from build123d import *

# Parameters (mm, degrees)
BASPROSKE_W         = 3
BASPROSKE_H         = 24.5
TOOTHCUT_DEPTH      = 35.777866525
TEETHCUTS_COUNT     = 26
TEETHCUTS_ANGLE     = 346.153846154
BORSKE_R            = 3
BORE_DEPTH          = 50.0000508
BOSS_EXTRUDE1_START = 3
SKETCH1_R           = 2.770499524
SKETCH1_R_2         = 3
BOSS_EXTRUDE1_DEPTH = 3


with BuildPart() as part:
    # BasProSke → Base-Revolve (revolve)
    with BuildSketch(Plane(origin=(0, 0, 0), x_dir=(1, 0, 0), z_dir=(0, 1, 0)), mode=Mode.PRIVATE) as base_revolve_sk:
        with Locations((1.5, 12.25)):
            Rectangle(BASPROSKE_W, BASPROSKE_H)
    revolve(base_revolve_sk.sketch.rotate(Axis((-10, 0, 0), (1, 0, 0)), 180), axis=Axis((-10, 0, 0), (1, 0, 0)))

    # TooCutSke → ToothCut (cut, through all)
    with BuildSketch(Plane(origin=(0, 0, 0), x_dir=(0, 0, -1), z_dir=(1, 0, 0))):
        with BuildLine():
            ThreePointArc((0.813448928, 20.545402967), (0, 20.5615), (-0.813448928, 20.545402967))
            ThreePointArc((-0.813448928, 20.545402967), (-1.408477569, 22.569593712), (-2.4536582, 24.402352481))
            ThreePointArc((-2.4536582, 24.402352481), (0, 24.5254), (2.4536582, 24.402352481))
            ThreePointArc((2.4536582, 24.402352481), (1.408477569, 22.569593712), (0.813448928, 20.545402967))
        make_face()
    toothcut = extrude(amount=TOOTHCUT_DEPTH, mode=Mode.SUBTRACT)

    # TeethCuts: ToothCut ×26 about axis
    teethcuts_axis = Axis((-10, 0, 0), (1, 0, 0))
    for i in range(1, TEETHCUTS_COUNT):
        add(toothcut.rotate(teethcuts_axis, i * TEETHCUTS_ANGLE / (TEETHCUTS_COUNT - 1)), mode=Mode.SUBTRACT)

    # BorSke → Bore (cut, symmetric)
    with BuildSketch(Plane(origin=(0, 0, 0), x_dir=(0, 0, -1), z_dir=(1, 0, 0))):
        with Locations(Location((0, 0, 0), (0, 0, 180))):
            Circle(BORSKE_R)
    extrude(amount=BORE_DEPTH, both=True, mode=Mode.SUBTRACT)

    # Sketch1 → Boss-Extrude1 (add)
    with BuildSketch(Plane(origin=(0, 0, 0), x_dir=(0, 0, -1), z_dir=(1, 0, 0)).offset(BOSS_EXTRUDE1_START)):
        with BuildLine():
            Line((-0.723220082, -5.956253245), (-54.329499283, 0.552727489))
            ThreePointArc((-54.329499283, 0.552727489), (-59.562532446, 7.232200815), (-52.88305912, 12.465233978))
            Line((-52.88305912, 12.465233978), (0.723220082, 5.956253245))
            ThreePointArc((0.723220082, 5.956253245), (5.956253245, -0.723220082), (-0.723220082, -5.956253245))
        make_face()
        with Locations((-53.606279201, 6.508980734)):
            Circle(SKETCH1_R, mode=Mode.SUBTRACT)
        with Locations(Location((0, 0, 0), (0, 0, 180))):
            Circle(SKETCH1_R_2, mode=Mode.SUBTRACT)
    extrude(amount=-BOSS_EXTRUDE1_DEPTH)


solid = part.part
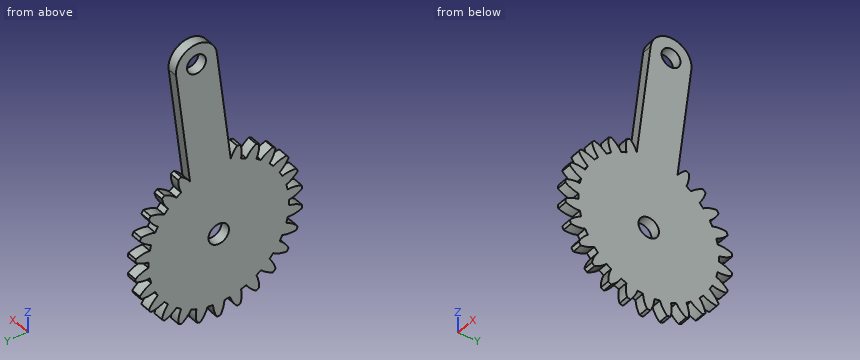
The listing builds one solid part. Answer for the finished solid, in the listing's coordinates (mm). Coordinates: 2 decimals unless noted, no trailing zeros. Write each loop counter-clockwise with the first axis right and the second up, starting at its lowest first coordinate (ties: lowest second). Pieces come first, ordered by that corner, then holes. Notation, with made-up numbers: (5, 18) - (54, 18) arc R32 cw to (54, 55) - close; hole circle Ø4 at (-13, 47.25). An arc over 180 degrees is marked (long way). Return JSON: item names as keys, results as strings.
1. Each of these flat-tipped pins is pushed along its axis until it touches: pin 1 Ø8 at (y, z) = (0, 0) entering from +X; pin 2 Ø1 at (x, z) = (2, 28.5) entering from -Y; pin 3 Ø1 at (y, z) = (-18.5, 17) entering from +X. Where does it stop, or does it pass through?
Final values:
{"pin 1": "x = 3", "pin 2": "y = -2.64", "pin 3": "through"}
2. The part is cut by section B-B on x = 0.95. Count the separate pieces of the cut face and the enclosed holes in it, then the cut area to 3 significant figures.
Final values:
{"separate pieces": "1", "enclosed holes": "2", "area": "1,980 mm^2"}
3. The part is cut by section A-A on z = 0. Determine the outline of the cut face in (x, y), then the cut area to 3 significant figures.
Final values:
{"outline": "(0, -20.56) - (3, -20.56) - (3, -3) - (0, -3) - close; (0, 3) - (3, 3) - (3, 20.56) - (0, 20.56) - close", "area": "105 mm^2"}
4. The part is cut by section C-C on z = 31. Determine the outline of the cut face in (x, y), then the cut area to 3 significant figures.
Final values:
{"outline": "(0, -2.28) - (3, -2.28) - (3, 9.81) - (0, 9.81) - close", "area": "36.3 mm^2"}
5. Consider line 1 along Z through (x, y) = (1.9, -22); line 2 along Z through (x, y) = (1.25, 15); line 3 along Y through (x, z) = (1.8, 0). Determine where each line is inside the solid, lowest interval first.
Final values:
{"line 1": "-9.25 to -7.11, -4.07 to -1.19, 1.19 to 4.07, 7.11 to 9.25", "line 2": "-18.33 to -14.44, -14.06 to 14.06, 14.44 to 18.33", "line 3": "-20.56 to -3, 3 to 20.56"}
